from build123d import *

# Parameters (mm, degrees)
SKETCH024_R  = 1.9
PAD015_DEPTH = 6
PAD016_DEPTH = 6


with BuildPart() as pad016:
    # Sketch024 → Pad015 (new body)
    with BuildSketch(Plane(origin=(-37, 0, 0), x_dir=(0, 1, 0), z_dir=(-1, 0, 0))):
        Polygon((46, 17), (40, 17), (40, 41), (26, 41), (26, 49), (46, 49), align=None)
        with Locations((43, 21)):
            Circle(SKETCH024_R, mode=Mode.SUBTRACT)
        with Locations((30, 45)):
            Circle(SKETCH024_R, mode=Mode.SUBTRACT)
        with Locations((43, 45)):
            Circle(SKETCH024_R, mode=Mode.SUBTRACT)
    extrude(amount=PAD015_DEPTH)

    # Sketch025 → Pad016 (new body)
    with BuildSketch(Plane(origin=(-37, 40, 0), x_dir=(0, 0, 1), z_dir=(0, -1, 0))):
        with BuildLine():
            Line((-41, 6), (-17, 6))
            ThreePointArc((-22.999973, 0), (-18.75735, 1.757369), (-17, 6))
            Line((-22.999973, 0), (-41, 0))
            Line((-41, 0), (-41, 6))
        make_face()
    extrude(amount=PAD016_DEPTH)


with BuildPart() as part_mirroring001:
    # Part__Mirroring001: instance of Pad016
    add(pad016.part.mirror(Plane(origin=(0, 0, 0), x_dir=(0, -1, 0), z_dir=(1, 0, 0))))


solid = part_mirroring001.part
Model file for the job. Use its own axes, mm. A direction names the side the tool comes from. Coordinates: 2 decimals unless noted, no trailing zeros. Order: outer loops, then holes, each group sorted by start corner. A loop starts at its lowest first (then second) coordinate and runs counter-clockwise, first axis right, second up. Notation, with made-up numbers: (-31, 17) -> (4, 17) arc R11 ccw to (4, 33) -> close; hole circle Ø10 at (-38, -0.5). An arc over 180 degrees is marked (long way). Return JSON: item names as keys, results as strings. Group by question number.
Item 1: Saw through at B-B on y = 30. Write the cut outline in (x, z).
Item 2: Saw through at A-A on z = -45. Write the cut outline in (x, y).
Item 3: Tool access for faces 1 (the cylindrical face through (38.711, 37.042, -18.804)), 2 (the flat face through (40, 30, -41)), 3 (the flat face through (40, 43, -17)): list every direction of +Z, -Z, +X, -X, +Y, -Y with a clear straight run to the whole face (end or side of a thin tool).
Item 4: Wall check: line 1 along Y through (x, z) = (38.35, -45); line 2 along Z through (x, y) = (39.3, 43); line 3 along Z through (x, y) = (39.5, 42.5). Give the ranges that are in metal, low to high. Write a range as [from, to].
Item 5: Flat gauge pins, fed straight in: P1, Ø3, axis at y = 43, z = -21, coming from the +X side; P2, Ø3, axis at x = 38.5, z = -20.5, coming from the -Y side. Where does each tip first touch, or does it go through?
Item 6: Saw through at D-D on x = 39.4. Write the cut outline in (y, z).
Item 7: Saw through at C-C on y = 43. Write the cut outline in (x, z).
Values found:
{
 "1": {"outline": "(37, -49) -> (43, -49) -> (43, -46.9) -> (37, -46.9) -> close; (37, -43.1) -> (43, -43.1) -> (43, -41) -> (37, -41) -> close"},
 "2": {"outline": "(37, 26) -> (43, 26) -> (43, 28.1) -> (37, 28.1) -> close; (37, 31.9) -> (43, 31.9) -> (43, 41.1) -> (37, 41.1) -> close; (37, 44.9) -> (43, 44.9) -> (43, 46) -> (37, 46) -> close"},
 "3": {"face 1": "+Z, -X, -Y", "face 2": "+Z, +X, -X, -Y", "face 3": "+Z, +X, -X, +Y, -Y"},
 "4": {"line 1": "y = [26, 28.1], [31.9, 41.1], [44.9, 46]", "line 2": "z = [-49, -46.9], [-43.1, -22.9], [-19.1, -17]", "line 3": "z = [-49, -46.83], [-43.17, -22.83], [-19.17, -17]"},
 "5": {"P1": "passes through", "P2": "stops at y = 34"},
 "6": {"outline": "(26, -49) -> (46, -49) -> (46, -17) -> (40, -17) -> (40, -18.2) -> (34, -18.2) -> (34, -41) -> (26, -41) -> close; hole circle Ø3.8 at (30, -45); hole circle Ø3.8 at (43, -45); hole circle Ø3.8 at (43, -21)"},
 "7": {"outline": "(37, -49) -> (43, -49) -> (43, -46.9) -> (37, -46.9) -> close; (37, -43.1) -> (43, -43.1) -> (43, -22.9) -> (37, -22.9) -> close; (37, -19.1) -> (43, -19.1) -> (43, -17) -> (37, -17) -> close"}
}
